CAD build for the part. Positions are in the model's coordinates, mm. A direction names the side the tool comes from. Give positions to 0.01 mm unless a question says otherwise; leave off trailing zeros. Loops run counter-clockwise (first coordinate to the right, second up) from the corner with the lowest first, then second, coordinate; pieces in that order, holes last.
```python
from build123d import *

# Parameters (mm, degrees)
SKETCH1_R           = 20
BOSS_EXTRUDE1_DEPTH = 13
SKETCH2_R           = 30
BOSS_EXTRUDE2_DEPTH = 8
SKETCH3_R           = 20
BOSS_EXTRUDE3_DEPTH = 13
CUT_EXTRUDE1_REACH  = 36
SKETCH4_R           = 12
SKETCH5_R           = 15.05
CUT_EXTRUDE2_DEPTH  = 2.4
CHAMFER1_SIZE       = 0.5
FILLET1_R           = 0.6
FILLET2_R           = 0.2
FILLET3_R           = 1


with BuildPart() as part:
    # Sketch1 → Boss-Extrude1 (new body)
    with BuildSketch(Plane.XY):
        Circle(SKETCH1_R)
    extrude(amount=BOSS_EXTRUDE1_DEPTH)

    # Sketch2 → Boss-Extrude2 (add)
    with BuildSketch(Plane(origin=(0, 0, 0), x_dir=(-1, 0, 0), z_dir=(0, 0, -1))):
        Circle(SKETCH2_R)
    extrude(amount=BOSS_EXTRUDE2_DEPTH)

    # Sketch3 → Boss-Extrude3 (add)
    with BuildSketch(Plane(origin=(0, 0, -8), x_dir=(-1, 0, 0), z_dir=(0, 0, -1))):
        Circle(SKETCH3_R)
    extrude(amount=BOSS_EXTRUDE3_DEPTH)

    # Sketch4 → Cut-Extrude1 (cut, up to next)
    with BuildSketch(Plane.XY.offset(13), mode=Mode.PRIVATE) as cut_extrude1_sk1:
        Circle(SKETCH4_R)
    cut_extrude1_tool1 = extrude(cut_extrude1_sk1.sketch, amount=-CUT_EXTRUDE1_REACH, mode=Mode.PRIVATE) & part.part
    add(cut_extrude1_tool1.solids().sort_by_distance((0, 0, 13))[0], mode=Mode.SUBTRACT)

    # Sketch5 → Cut-Extrude2 (cut)
    with BuildSketch(Plane.XY.offset(13)):
        Circle(SKETCH5_R)
    extrude(amount=-CUT_EXTRUDE2_DEPTH, mode=Mode.SUBTRACT)

    # Chamfer1
    chamfer1_edges = [part.edges().sort_by_distance(p)[0] for p in [
        (20, 0, -21),
        (-12, 0, -21),
        (-20, 0, 13),
        (30, 0, 0),
        (30, 0, -8),
    ]]
    chamfer(chamfer1_edges, length=CHAMFER1_SIZE)

    # Fillet1
    fillet1_edges = [part.edges().sort_by_distance(p)[0] for p in [
        (-20, 0, 0),
        (20, 0, -8),
    ]]
    fillet(fillet1_edges, radius=FILLET1_R)

    # Fillet2
    fillet2_edges = [part.edges().sort_by_distance(p)[0] for p in [
        (-15.05, 0, 13),
        (-12, 0, 10.6),
    ]]
    fillet(fillet2_edges, radius=FILLET2_R)

    # Fillet3
    fillet3_edges = [part.edges().sort_by_distance(p)[0] for p in [
        (-15.05, 0, 10.6),
    ]]
    fillet(fillet3_edges, radius=FILLET3_R)


solid = part.part
```
1. Pull direction Y, two halves, no side cores. Call faces 1 (the face through (4.336, -19.524, -14.467)), 2 (the face through (-4, 12, 10.6)), 3 (the face through (20, -6, -8)): released by +Y, released by -Y, zero draft, split by the parting line, or undercut.
Responses:
face 1: split by the parting line
face 2: undercut
face 3: zero draft
2. Drop flat-ended pins along their axis: pin 1 (6 mm diameter, centred on x = -20, z = -0.5, fed in from +Y); pin 2 (5 mm diameter, centred on x = -19, z = 8, fed in from -Y); pin 3 (1 mm diameter, centred on y = -14, z = 2, fed in from +X); pin 4 (8.5 mm diameter, centred on x = 4.5, y = -1, fed in from +Z). Give the stop position or say it passes through.
Responses:
pin 1: stops at y = 24.72
pin 2: stops at y = -11.3
pin 3: stops at x = 14.76
pin 4: passes through
3. Saw through at B-B, the plane z = -17. List the corners of the cut face in (x, y), and give its area (3 significant figures).
Responses:
outline: circle Ø40 at (0, 0); hole circle Ø24 at (0, 0)
area: 804 mm2
4. Probe line 1 along Y through (x, z) = (0, -11); line 2 along Y through (x, z) = (0, 12.4); line 3 along Y through (x, z) = (26.5, -4.5). List the from-to ranges inside material, lowest first.
Responses:
line 1: y = -20 to -12, 12 to 20
line 2: y = -20 to -15.05, 15.05 to 20
line 3: y = -14.06 to 14.06
5. Saw through at A-A, the plane z = -3.5. List the corners of the cut face in (x, y).
Responses:
outline: circle Ø60 at (0, 0); hole circle Ø24 at (0, 0)
6. Tool access for faces 4 (the face through (29.97, 1.32, -3.95)), 5 (the face through (-3.263, -14.692, 12.208)): list every direction of +Z, -Z, +X, -X, +Y, -Y with a clear straight run to the whole face (end or side of a thin tool).
Responses:
face 4: +Z, -Z
face 5: +Z
